from build123d import *

# Parameters (mm, degrees)
BOSS_EXTRUDE1_DEPTH                             = 27.5
SKETCH4_W                                       = 45
SKETCH4_H                                       = 9.976183447
BOSS_EXTRUDE2_DEPTH                             = 4.5
CSK_FOR_M5_FLAT_HEAD_MACHINE_SCREW1_AT_2_COUNT  = 2
CSK_FOR_M5_FLAT_HEAD_MACHINE_SCREW1_AT_2_PITCH  = 32
CSK_FOR_M5_FLAT_HEAD_MACHINE_SCREW1_AT_3_COUNT  = 2
CSK_FOR_M5_FLAT_HEAD_MACHINE_SCREW1_AT_3_PITCH  = 43.863424399
CSK_FOR_M5_FLAT_HEAD_MACHINE_SCREW1_AT_4_COUNT  = 2
CSK_FOR_M5_FLAT_HEAD_MACHINE_SCREW1_AT_4_PITCH  = 30
CUT_EXTRUDE1_REACH                              = 136.892
CUT_EXTRUDE1_END_RADIUS                         = 57.15
SKETCH13_R                                      = 5.2
CHAMFER1_SIZE                                   = 3.142829186
CHAMFER1_SIZE_2                                 = 3.175
CHAMFER2_SIZE                                   = 1
CSK_FOR_M3_FLAT_HEAD_MACHINE_SCREW1_D           = 3.4
CSK_FOR_M3_FLAT_HEAD_MACHINE_SCREW1_DEPTH       = 15
CSK_FOR_M3_FLAT_HEAD_MACHINE_SCREW1_CSINK_D     = 6.3
CSK_FOR_M3_FLAT_HEAD_MACHINE_SCREW1_CSINK_ANGLE = 90
CSK_FOR_M3_FLAT_HEAD_MACHINE_SCREW1_TIP         = 1.021463052
FILLET2_R                                       = 5
SKETCH14_R                                      = 3.175
CUT_EXTRUDE2_DEPTH                              = 10


with BuildPart() as part:
    # Sketch1 → Boss-Extrude1 (new, symmetric)
    with BuildSketch(Plane(origin=(0, 0, 0), x_dir=(1, 0, 0), z_dir=(0, 1, 0))):
        with BuildLine():
            Line((-27.5, 53.692230583), (-27.5, 72.301183447))
            Line((-27.5, 72.301183447), (-22.5, 72.301183447))
            Line((-22.5, 72.301183447), (-22.5, 62.325))
            Line((-22.5, 62.325), (22.5, 62.325))
            Line((22.5, 62.325), (22.5, 72.301183447))
            Line((22.5, 72.301183447), (27.5, 72.301183447))
            Line((27.5, 72.301183447), (32.466110956, 68.134121575))
            Line((32.466110956, 68.134121575), (23.851795776, 57.867980511))
            Line((23.851795776, 57.867980511), (27.682017991, 54.654042463))
            Line((27.682017991, 54.654042463), (36.296333172, 64.920183527))
            Line((36.296333172, 64.920183527), (40.126555387, 61.706245479))
            Line((40.126555387, 61.706245479), (31.512240207, 51.440104414))
            Line((31.512240207, 51.440104414), (33.340523926, 46.41693618))
            ThreePointArc((33.340523926, 46.41693618), (-34.836825197, -45.304725032), (36.296051801, 44.144298881))
            Line((36.296051801, 44.144298881), (34.301778965, 49.623518465))
            Line((34.301778965, 49.623518465), (42.658017891, 59.582096225))
            Line((42.658017891, 59.582096225), (46.488240107, 56.368158177))
            Line((46.488240107, 56.368158177), (38.298629476, 46.608160286))
            ThreePointArc((38.298629476, 46.608160286), (25.775383623, -54.541133322), (-60.325, 0))
            Line((-60.325, 0), (-60.325, 92.301183447))
            Line((-60.325, 92.301183447), (-52.325, 92.301183447))
            Line((-52.325, 92.301183447), (-52.325, 30.019993338))
            ThreePointArc((-52.325, 30.019993338), (-41.63053399, 43.657808748), (-27.5, 53.692230583))
        make_face()
    extrude(amount=BOSS_EXTRUDE1_DEPTH, both=True)

    # Sketch4 → Boss-Extrude2 (add)
    with BuildSketch(Plane.XZ.offset(27.5)):
        with Locations((0, -67.313091724)):
            Rectangle(SKETCH4_W, SKETCH4_H)
    extrude(amount=-BOSS_EXTRUDE2_DEPTH)

    # Sketch12 → CSK for M5 Flat Head Machine Screw1 (revolve, cut)
    with BuildSketch(Plane(origin=(-16, 15, -57.15), x_dir=(0, -1, 0), z_dir=(1, 0, 0))):
        Polygon((0, 0), (0, 35.151183447), (2.75, 35.151183447), (2.75, 2.45), (5.2, 0), align=None)
    csk_for_m5_flat_head_machine_screw1 = revolve(axis=Axis((-16, 15, -50.8), (0, 0, -1)), mode=Mode.SUBTRACT)

    # CSK for M5 Flat Head Machine Screw1 at 2: CSK for M5 Flat Head Machine Screw1 ×2
    with Locations(*[(i * CSK_FOR_M5_FLAT_HEAD_MACHINE_SCREW1_AT_2_PITCH, 0, 0) for i in range(1, CSK_FOR_M5_FLAT_HEAD_MACHINE_SCREW1_AT_2_COUNT)]):
        add(csk_for_m5_flat_head_machine_screw1, mode=Mode.SUBTRACT)

    # CSK for M5 Flat Head Machine Screw1 at 3: CSK for M5 Flat Head Machine Screw1 ×2
    with Locations(*[Vector(0.7295372041400852, -0.6839411288813297, 0) * (i * CSK_FOR_M5_FLAT_HEAD_MACHINE_SCREW1_AT_3_PITCH) for i in range(1, CSK_FOR_M5_FLAT_HEAD_MACHINE_SCREW1_AT_3_COUNT)]):
        add(csk_for_m5_flat_head_machine_screw1, mode=Mode.SUBTRACT)

    # CSK for M5 Flat Head Machine Screw1 at 4: CSK for M5 Flat Head Machine Screw1 ×2
    with Locations(*[(0, -i * CSK_FOR_M5_FLAT_HEAD_MACHINE_SCREW1_AT_4_PITCH, 0) for i in range(1, CSK_FOR_M5_FLAT_HEAD_MACHINE_SCREW1_AT_4_COUNT)]):
        add(csk_for_m5_flat_head_machine_screw1, mode=Mode.SUBTRACT)

    # Cut-Extrude1: up to this cylinder (the profile starts outside it)
    cut_extrude1_end = Plane(origin=(0, 0, 0), z_dir=(0, -1, 0)) * Cylinder(CUT_EXTRUDE1_END_RADIUS, 419.084, mode=Mode.PRIVATE)
    # Sketch13 → Cut-Extrude1 (cut, up to the surface)
    with BuildSketch(Plane.XY.offset(-57.15), mode=Mode.PRIVATE) as cut_extrude1_sk1:
        with Locations(Location((-16, -15, 0), (0, 0, 180))):
            Circle(SKETCH13_R)
    cut_extrude1_tool1 = extrude(cut_extrude1_sk1.sketch, amount=CUT_EXTRUDE1_REACH, mode=Mode.PRIVATE) - cut_extrude1_end
    add(cut_extrude1_tool1.solids().sort_by_distance((-16, -15, -57.15))[0], mode=Mode.SUBTRACT)
    # Sketch13 → Cut-Extrude1 (cut, up to the surface)
    with BuildSketch(Plane.XY.offset(-57.15), mode=Mode.PRIVATE) as cut_extrude1_sk2:
        with Locations(Location((16, -15, 0), (0, 0, 180))):
            Circle(SKETCH13_R)
    cut_extrude1_tool2 = extrude(cut_extrude1_sk2.sketch, amount=CUT_EXTRUDE1_REACH, mode=Mode.PRIVATE) - cut_extrude1_end
    add(cut_extrude1_tool2.solids().sort_by_distance((16, -15, -57.15))[0], mode=Mode.SUBTRACT)
    # Sketch13 → Cut-Extrude1 (cut, up to the surface)
    with BuildSketch(Plane.XY.offset(-57.15), mode=Mode.PRIVATE) as cut_extrude1_sk3:
        with Locations(Location((16, 15, 0), (0, 0, 180))):
            Circle(SKETCH13_R)
    cut_extrude1_tool3 = extrude(cut_extrude1_sk3.sketch, amount=CUT_EXTRUDE1_REACH, mode=Mode.PRIVATE) - cut_extrude1_end
    add(cut_extrude1_tool3.solids().sort_by_distance((16, 15, -57.15))[0], mode=Mode.SUBTRACT)
    # Sketch13 → Cut-Extrude1 (cut, up to the surface)
    with BuildSketch(Plane.XY.offset(-57.15), mode=Mode.PRIVATE) as cut_extrude1_sk4:
        with Locations(Location((-16, 15, 0), (0, 0, 180))):
            Circle(SKETCH13_R)
    cut_extrude1_tool4 = extrude(cut_extrude1_sk4.sketch, amount=CUT_EXTRUDE1_REACH, mode=Mode.PRIVATE) - cut_extrude1_end
    add(cut_extrude1_tool4.solids().sort_by_distance((-16, 15, -57.15))[0], mode=Mode.SUBTRACT)

    # Chamfer1
    # the kernel refuses this chamfer: 7.31254539, 3.175, 3.142829186 mm, written as the material it adds along each edge
    with BuildSketch(Plane(origin=(38.298629476, 27.5, -46.608160286), x_dir=(0.6427876096865355, 0, -0.7660444431189813), z_dir=(0, -1, 0))) as chamfer1_piece_1:
        with BuildLine():
            Line((CHAMFER1_SIZE, 0), (-0.054749246, 3.264067078))
            ThreePointArc((-0.054749246, 3.264067078), (-0.006082575, 1.678547233), (0, 0))
            Line((0, 0), (CHAMFER1_SIZE, 0))
        make_face()
    extrude(amount=55)
    with BuildSketch(Plane(origin=(-27.5, -27.5, -53.692230583), x_dir=(0, 0, -1), z_dir=(0, 1, 0))) as chamfer1_piece_2:
        with BuildLine():
            Line((CHAMFER1_SIZE_2, 0), (-5.17652137, 8.35152137))
            ThreePointArc((-5.17652137, 8.35152137), (-2.493388985, 4.40273098), (0, 0))
            Line((0, 0), (CHAMFER1_SIZE_2, 0))
        make_face()
    extrude(amount=55)

    # Chamfer2
    chamfer2_edges = [part.edges().sort_by_distance(p)[0] for p in [
        (23.851795776, 0, -57.867980511),
        (27.682017991, 0, -54.654042463),
    ]]
    chamfer(chamfer2_edges, length=CHAMFER2_SIZE)

    # CSK for M3 Flat Head Machine Screw1
    with Locations(Plane(origin=(-0.475480456, 0, -0.398975475), x_dir=(0.6427876096865344, 0, -0.7660444431189822), z_dir=(0.7660444431189822, 0, 0.6427876096865344))):
        with Locations((68.263607475, 20), (68.263607475, 0), (68.263607475, -20)):
            CounterSinkHole(CSK_FOR_M3_FLAT_HEAD_MACHINE_SCREW1_D / 2, CSK_FOR_M3_FLAT_HEAD_MACHINE_SCREW1_CSINK_D / 2, depth=CSK_FOR_M3_FLAT_HEAD_MACHINE_SCREW1_DEPTH, counter_sink_angle=CSK_FOR_M3_FLAT_HEAD_MACHINE_SCREW1_CSINK_ANGLE)
            with Locations((0, 0, -(CSK_FOR_M3_FLAT_HEAD_MACHINE_SCREW1_DEPTH + CSK_FOR_M3_FLAT_HEAD_MACHINE_SCREW1_TIP / 2))):  # 118° drill point
                Cone(0, CSK_FOR_M3_FLAT_HEAD_MACHINE_SCREW1_D / 2, CSK_FOR_M3_FLAT_HEAD_MACHINE_SCREW1_TIP, mode=Mode.SUBTRACT)

    # Fillet2
    fillet2_edges = [part.edges().sort_by_distance(p)[0] for p in [
        (-52.325, 0, -30.019993338),
    ]]
    fillet(fillet2_edges, radius=FILLET2_R)

    # Sketch14 → Cut-Extrude2 (cut)
    with BuildSketch(Plane(origin=(-52.325, 0, 0), x_dir=(0, 0, -1), z_dir=(1, 0, 0))):
        with Locations((84.301183447, 12.7)):
            Circle(SKETCH14_R)
        with Locations((84.301183447, -12.7)):
            Circle(SKETCH14_R)
    extrude(amount=-CUT_EXTRUDE2_DEPTH, mode=Mode.SUBTRACT)


solid = part.part
The model under review builds one solid part; all positions refer to its coordinate system, in mm. A direction names the side the tool comes from. Round coordinates to 2 decimals unless told otherwise and drop trailing zeros. Loops run counter-clockwise (first coordinate to the right, second up) from the corner with the lowest first, then second, coordinate; pieces in that order, holes last. Notation, with made-up numbers: (-20.5, -22.5) -> (-5.5, -22.5) arc R9 ccw to (-5.5, -11.5) -> close; hole circle Ø11 at (25, 71). An arc over 180 degrees is marked (long way). Return JSON: item names as keys, results as strings.
(1) Add section B-B on z = -8.5. Write out the cut boundary in (x, y) (3 decimals).
Solved:
{"outline": "(-60.325, -27.5) -> (-56.514, -27.5) -> (-56.514, 27.5) -> (-60.325, 27.5) -> close; (56.514, -27.5) -> (59.723, -27.5) -> (59.723, 27.5) -> (56.514, 27.5) -> close"}
(2) Add section A-A on x = -16. Write out the cut boundary in (y, z) (3 decimals), plus the area to 3 significant figures.
Solved:
{"outline": "(-27.5, -72.301) -> (-23, -72.301) -> (-23, -62.325) -> (-17.75, -62.325) -> (-17.75, -59.6) -> (-20.2, -57.15) -> (-20.2, -54.865) -> (-27.5, -54.865) -> close; (-27.5, 54.865) -> (27.5, 54.865) -> (27.5, 58.164) -> (-27.5, 58.164) -> close; (-12.25, -62.325) -> (12.25, -62.325) -> (12.25, -59.6) -> (9.8, -57.15) -> (9.8, -54.865) -> (-9.8, -54.865) -> (-9.8, -57.15) -> (-12.25, -59.6) -> close; (17.75, -62.325) -> (27.5, -62.325) -> (27.5, -54.865) -> (20.2, -54.865) -> (20.2, -57.15) -> (17.75, -59.6) -> close", "area": "520 mm2"}
(3) For pin 1 (1 mm diameter, centred on x = -11.5, y = -3.5, fed in from +Z); pin 2 (8.5 mm diameter, centred on y = -12.7, z = -84.3, fed in from +X) (3 decimals); pin 3 (9 mm diameter, centred on x = -16, y = -15, fed in from +Z), all flat-tipped, find the tip position at first contact; note any pin that passes through.
Solved:
{"pin 1": "z = 59.31", "pin 2": "x = -52.325", "pin 3": "z = 59.22"}
(4) The part is to be moulded in two halves that separate along Z. For faces 6 (the cylindrical face through (-56.27, -14.63, -81.78)), 7 (the flat face through (22.5, 3, -67)), 8 (the flat face through (-56, 0, -92.301)), say which applies: released by +Z, released by -Z, zero draft, split by the parting line, or undercut.
Solved:
{"face 6": "undercut", "face 7": "zero draft", "face 8": "released by -Z"}
(5) For faces 1 (the flat face through (37.493, 0.385, -53.427)), 2 (the cylindrical face through (21.195, -15.229, -55.593)), 3 (the cylindrical face through (-39.983, 0.385, -45.172)), 4 (the flat face through (-22.5, 3, -67)), 5 (the flat face through (40.705, 0.385, -49.476)), list the 3-axis set-ups (+Z, -Z, +X, -X, +Y, -Y) from which the entire face can be reached by the end or side of a thin tool; tool diameter is ignored.
Solved:
{"face 1": "+Y, -Y", "face 2": "none", "face 3": "-Z, +Y, -Y", "face 4": "-Z, +Y", "face 5": "+X, +Y, -Y"}
(6) Add section C-C on y = 5. Write out the cut boundary in (x, z) (3 decimals).
Solved:
{"outline": "(-60.325, -92.301) -> (-52.325, -92.301) -> (-52.325, -45.03) arc R5 cw to (-43.703, -41.583) arc R60.325 ccw to (-35.852, -48.516) -> (-27.5, -56.867) -> (-27.5, -72.301) -> (-22.5, -72.301) -> (-22.5, -62.325) -> (22.5, -62.325) -> (22.5, -72.301) -> (27.5, -72.301) -> (32.466, -68.134) -> (24.495, -58.634) -> (24.618, -57.225) -> (26.916, -55.297) -> (28.325, -55.42) -> (36.296, -64.92) -> (40.127, -61.706) -> (31.512, -51.44) -> (33.341, -46.417) arc R57.15 cw (long way) to (36.296, -44.144) -> (34.302, -49.624) -> (42.658, -59.582) -> (46.488, -56.368) -> (40.319, -49.016) -> (40.764, -44.468) arc R60.325 ccw (long way) to (-60.325, 0) -> close"}
(7) Add section D-D on x = -0.5. Write out the cut boundary in (y, z) (3 decimals), plus the area to 3 significant figures.
Solved:
{"outline": "(-27.5, -72.301) -> (-23, -72.301) -> (-23, -62.325) -> (27.5, -62.325) -> (27.5, -57.148) -> (-27.5, -57.148) -> close; (-27.5, 57.148) -> (27.5, 57.148) -> (27.5, 60.323) -> (-27.5, 60.323) -> close", "area": "504 mm2"}
(8) For line 1 (Y direction, x = 16, z = -55.4); line 2 (X direction, y = -15, z = -60.55) (3 decimals); line 3 (Z direction, x = -43.5, y = -24.5), list the stretches that pass through material, from the lowest coordinate up.
Solved:
{"line 1": "-27.5 to -20.2, -9.8 to 9.8, 20.2 to 27.5", "line 2": "-60.325 to -52.325, -27.5 to -18.75, -13.25 to 13.25, 18.75 to 26.102, 32.629 to 39.156", "line 3": "-41.8 to -37.07, 37.07 to 41.8"}
